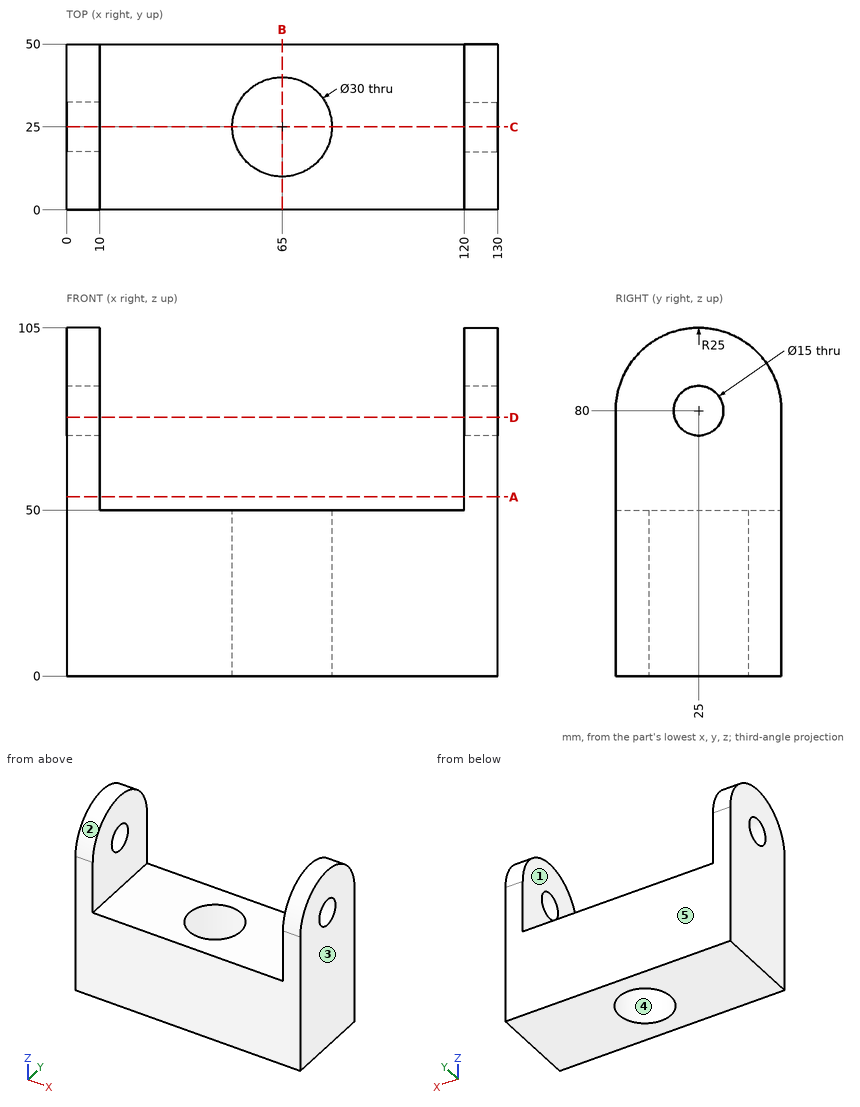
Could you check a few things on this drawing? It's one solid part, dimensions in mm from its lowest x, y, z. A direction names the side the tool comes from. Give positions to 0.01 mm unless a question says otherwise; leave off trailing zeros. Order: outer loops, then holes, each group sorted by start corner. A loop starts at its lowest first (then second) coordinate and runs counter-clockwise, first axis right, second up. Notation, with made-up numbers: (9.5, 3.25) -> (67.5, 3.25) arc R29 ccw to (67.5, 37.25) -> close; hole circle Ø4 at (8, -40). An arc over 180 degrees is marked (long way). Answer in a Markdown table with one row per item. Add a question column.
Item 1: We'd pull the mould along X, two halves only. Please class the marked faces 3, 4 and 5: pulls with the +X half, pulls with the -X half, needs draft (parallel to the pull), parting line crosses it, or undercut.
Item 2: Imagine slicing it at A-A (z = 54). List the corners of the cut face in (x, y) for me.
Item 3: I'm going to push flat-ended pins straight in: P1, Ø3, axis at y = 19.5, z = 66.5, coming from the -X side; P2, Ø4, axis at x = 34.5, y = 44.5, coming from the +Z side. Where does each tip first touch, or does it pass through?
Item 4: Imagine slicing it at D-D (z = 78). List the corners of the cut face in (x, y) for me.
Item 5: Imagine slicing it at B-B (x = 65). List the corners of the cut face in (y, z) for me.
Item 6: Please list where these lines run through material, in increasing order: probe 1 along Y at (x, z) = (127, 80); probe 2 along X at (y, z) = (33, 53.5); probe 3 along Y at (x, z) = (65, 19).
Item 7: Imagine slicing it at C-C (y = 25). List the corners of the cut face in (x, z) for me, and give its area (3 significant figures).
Item 8: For the marked faces 1 and 2, which set-ups out of +Z, -Z, +X, -X, +Y, -Y let a thin tool reach every point of the face, with its end or its side?
Result:
| question | item | result |
|---|---|---|
| 1 | face 3 | pulls with the +X half |
| 1 | face 4 | undercut |
| 1 | face 5 | needs draft |
| 2 | outline | (0, 0) -> (10, 0) -> (10, 50) -> (0, 50) -> close; (120, 0) -> (130, 0) -> (130, 50) -> (120, 50) -> close |
| 3 | P1 | x = 0 |
| 3 | P2 | z = 50 |
| 4 | outline | (0, 0) -> (10, 0) -> (10, 17.77) -> (0, 17.77) -> close; (0, 32.23) -> (10, 32.23) -> (10, 50) -> (0, 50) -> close; (120, 0) -> (130, 0) -> (130, 17.77) -> (120, 17.77) -> close; (120, 32.23) -> (130, 32.23) -> (130, 50) -> (120, 50) -> close |
| 5 | outline | (0, 0) -> (10, 0) -> (10, 50) -> (0, 50) -> close; (40, 0) -> (50, 0) -> (50, 50) -> (40, 50) -> close |
| 6 | probe 1 | 0 to 17.5, 32.5 to 50 |
| 6 | probe 2 | 0 to 10, 120 to 130 |
| 6 | probe 3 | 0 to 10, 40 to 50 |
| 7 | outline | (0, 0) -> (50, 0) -> (50, 50) -> (10, 50) -> (10, 72.5) -> (0, 72.5) -> close; (0, 87.5) -> (10, 87.5) -> (10, 105) -> (0, 105) -> close; (80, 0) -> (130, 0) -> (130, 72.5) -> (120, 72.5) -> (120, 50) -> (80, 50) -> close; (120, 87.5) -> (130, 87.5) -> (130, 105) -> (120, 105) -> close |
| 7 | area | 5,800 mm2 |
| 8 | face 1 | +Z, +Y, -Y |
| 8 | face 2 | +Z, +X, -X |
